The model under review builds one solid part; all positions refer to its coordinate system, in mm. Give positions to 0.01 mm unless a question says otherwise; leave off trailing zeros. Write each loop counter-clockwise with the first axis right and the second up, starting at its lowest first coordinate (ties: lowest second). Pieces come first, ordered by that corner, then holes. Notation, with made-up numbers: (-6, 25) - (11, 25) arc R7 cw to (11, 36) - close; hole circle Ø11 at (29, -20). An arc over 180 degrees is marked (long way). Write item = value, one per line.
Autodesk Inventor part; units mm, degrees
ref_plane "YZ Plane" through (0, 0, 0) normal (1, 0, 0) x (0, 1, 0)
ref_plane "XZ Plane" through (0, 0, 0) normal (0, 1, 0) x (-1, 0, 0)
ref_plane "XY Plane" through (0, 0, 0) normal (0, 0, 1) x (1, 0, 0)
sketch "Sketch1" plane through (0, 0, 0) normal (0, 0, 1) x (1, 0, 0)
  arc A0 (38.1, 0) -> (-38.1, 0) centre (0, 0) ccw
  arc A1 (50.8, 0) -> (-50.8, 0) centre (0, 0) ccw
  line L0 (-50.8, 0) -> (-38.1, 0)
  line L1 (38.1, 0) -> (50.8, 0)
  dimension "d0" = 76.2
  dimension "d1" = 12.7
extrude "Extrusion1" add sketch "Sketch1" along normal blind 24.13
sketch "Sketch2" plane through (38.1, 0, 0) normal (0, -1, 0) x (1, 0, 0)
  line L0 (12.7, 0) -> (12.7, 24.13) construction
  circle A0 centre (12.7, 12.065) radius 9.525
  point P0 (-38.1, 0)
  dimension "d4" = 19.05
extrude "Extrusion2" add sketch "Sketch2" against normal blind 15.25
sketch "Sketch3" plane through (38.1, 15.25, 0) normal (0, 1, 0) x (1, 0, 0)
  arc A0 (12.7, -21.59) -> (12.7, -2.54) centre (12.7, -12.065) ccw
  circle A1 centre (12.7, -12.065) radius 9.525
  point P0 (-38.1, 0)
  dimension "d7" = 19.05
extrude "Extrusion3" cut sketch "Sketch3" along normal blind 15.25 draft 3
sketch "Sketch4" plane through (38.1, 15.25, 0) normal (0, 1, 0) x (1, 0, 0)
  arc A0 (10.357, -21.2973) -> (10.357, -2.8327) centre (12.7, -12.065) ccw
  point P0 (-38.1, 0)
hole "Hole1" at (50.8, 15.25, 12.065) direction (0, -1, 0) diameter 8.433 end through all
mirror "Mirror1" about plane through (0, 0, 0) normal (1, 0, 0) of "Extrusion2", "Extrusion3", "Hole1"
fillet "Fillet1" radius 2.54 2 edges at (0, 50.8, 24.13) (0, 50.8, 0)
thread "Thread1"
thread "Thread2"
properties part number "Pistonhandattacher"
1. Insertion check: P1, Ø8, axis at x = -13, z = 18.5, coming from the -Y side; P2, Ø5.5, axis at x = -53.5, z = 15, coming from the +Y side; P3, Ø1.5, axis at x = -21.5, z = 17, coming from the +Y side. Each pin has a flat end and moves straight along its axis. Give the tip position at first contact, or say it passes through.
Findings below:
P1 = 34.1
P2 = 15.25
P3 = 46.37
2. Take a section at A-A on x = 0. Give the boundary of the cut face in (y, z).
Findings below:
outline = (38.1, 0) - (48.26, 0) arc R2.54 ccw to (50.8, 2.54) - (50.8, 21.59) arc R2.54 ccw to (48.26, 24.13) - (38.1, 24.13) - close
3. Draft analysis for pull direction Z (two halves, no side actions). For faces 1 (the flat face through (55, 15.25, 10)), 2 (the flat face through (3, 39, 0)), 3 (the flat face through (47, 0, 9)), state which applies: +Z half, -Z half, draft (parallel to the pull), parting line (faces both ways), or undercut.
Findings below:
face_1 = undercut
face_2 = -Z half
face_3 = draft
4. For line 1 (Z direction, x = -50.8, y = 11.5); line 2 (X direction, y = 23, z = 5.25); line 3 (X direction, y = 7.5, z = 13), list the stretches that pass through material, from the lowest coordinate up. Write a range as from..to.
Findings below:
line_1 = 2.54..7.85, 16.28..21.59
line_2 = -43.58..-30.37, 30.37..43.58
line_3 = -60.28..-54.91, -46.69..-37.35, 37.35..46.69, 54.91..60.28
